Here's how the part is built. I have some questions about the finished solid (model axes, mm). A direction names the side the tool comes from. Give positions to 0.01 mm unless a question says otherwise; leave off trailing zeros. Loops run counter-clockwise (first coordinate to the right, second up) from the corner with the lowest first, then second, coordinate; pieces in that order, holes last. Notation, with made-up numbers: (55, 64.25) - (65, 64.25) arc R24 cw to (65, 95.25) - close; hole circle Ø11 at (73, -7). An arc over 180 degrees is marked (long way). Use a Markdown table: item, result.
Autodesk Inventor part; units mm, degrees
ref_plane "YZ Plane" through (0, 0, 0) normal (1, 0, 0) x (0, 1, 0)
ref_plane "XZ Plane" through (0, 0, 0) normal (0, 1, 0) x (-1, 0, 0)
ref_plane "XY Plane" through (0, 0, 0) normal (0, 0, 1) x (1, 0, 0)
sketch "Sketch1" plane through (0, 0, 0) normal (0, 0, 1) x (1, 0, 0)
  circle A0 centre (0, 0) radius 50
  circle A1 centre (0, 0) radius 35
  line L0 (-20, 45) -> (20, 45)
  line L1 (20, 45) -> (20, -75)
  line L2 (20, -75) -> (-20, -75)
  line L3 (-20, -75) -> (-20, 45)
  line L4 (-32.4459, -13.125) -> (-32.4459, -38.0429)
  line L5 (32.4459, -13.125) -> (32.4459, -38.0429)
  line L6 (-10, -67) -> (10, -67)
  line L7 (10, -67) -> (10, -64)
  line L8 (10, -64) -> (-10, -64)
  line L9 (-10, -64) -> (-10, -67)
  dimension "d0" = 100
  dimension "d1" = 70
  dimension "d4" = 40
  dimension "d5" = 120
  dimension "d9" = 20
  dimension "d10" = 3
extrude "Extrusion2" add sketch "Sketch1" along normal blind 5.5 contours A0 L5 A1 L1 L0 L3 L4 | L3 A1 L1 A0 | A0 L1 L2 L3 | L3 A1 L1 | L3 L0 L1 A1 | L9 L8 L7 L6
fillet "Fillet1" radius 8 2 edges at (20, -75, 2.75) (-20, -75, 2.75)
sketch "Sketch2" plane through (0, 0, 5.5) normal (0, 0, 1) x (1, 0, 0)
  line L0 (-10, -67) -> (10, -67)
  line L1 (10, -67) -> (10, -64)
  line L2 (10, -64) -> (-10, -64)
  line L3 (-10, -64) -> (-10, -67)
  point P0 (0, 0)
  dimension "d11" = 20
  dimension "d12" = 3
extrude "Extrusion3" cut sketch "Sketch2" against normal blind 5.5
sketch "Sketch4" plane through (0, 0, 5.5) normal (0, 0, 1) x (1, 0, 0)
  line L0 (39.75, 2.75) -> (45.25, 2.75)
  line L1 (45.25, 2.75) -> (45.25, -2.75)
  line L2 (45.25, -2.75) -> (39.75, -2.75)
  line L3 (39.75, -2.75) -> (39.75, 2.75)
  line L4 (-39.75, -2.75) -> (-45.25, -2.75)
  line L5 (-45.25, -2.75) -> (-45.25, 2.75)
  line L6 (-45.25, 2.75) -> (-39.75, 2.75)
  line L7 (-39.75, 2.75) -> (-39.75, -2.75)
  point P0 (0, 0)
  point P1 (0, 0)
  dimension "d24" = 5.5
  dimension "d25" = 5.5
  dimension "d26" = 360
extrude "Extrusion5" cut sketch "Sketch4" against normal blind 10
properties part number "central"
(1) We'd pull the mould along X, two halves only. Please class faces 4 (the face through (-17.719, -72.594, 2.788)), 5 (the face through (33.452, 10.293, 2.712)), 6 (the face through (-1.7, 49.97, 2.71)), 7 (the face through (32.446, -25, 3)): pulls with the +X half, pulls with the -X half, needs draft (parallel to the pull), parting line crosses it, or undercut.
A:
| item | result |
|---|---|
| face 4 | pulls with the -X half |
| face 5 | undercut |
| face 6 | parting line crosses it |
| face 7 | undercut |
(2) Suppose I cut it at B-B on x = 0. Write out the boundary of the cut face in (y, z), plus the area to 3 significant figures.
A:
| item | result |
|---|---|
| outline | (-75, 0) - (-67, 0) - (-67, 5.5) - (-75, 5.5) - close; (-64, 0) - (50, 0) - (50, 5.5) - (-64, 5.5) - close |
| area | 671 mm2 |
(3) On a 3-axis mill with a long thin cutter (end or side, diameter ignored), from which of +Z, -Z, +X, -X, +Y, -Y can I reach the whole of each face in a straight line? I mean faces 1 (the face through (0, -67, 3)), 2 (the face through (-20, -20, 3)), 3 (the face through (17.594, -72.719, 2.788)). Say none if no direction works.
A:
| item | result |
|---|---|
| face 1 | +Z, -Z |
| face 2 | +Z, -Z, -Y |
| face 3 | +Z, -Z, +X, -Y |
(4) Suppose I cut it at D-D on z = 4.6. Write out the boundary of the cut face in (x, y) (3 decimals).
A:
| item | result |
|---|---|
| outline | (-32.446, -38.043) - (-32.446, -13.125) arc R35 cw to (-20, 28.723) - (-20, -67) arc R8 ccw to (-12, -75) - (12, -75) arc R8 ccw to (20, -67) - (20, 28.723) arc R35 cw to (32.446, -13.125) - (32.446, -38.043) arc R50 ccw (long way) to start; hole (-45.25, -2.75) - (-39.75, -2.75) - (-39.75, 2.75) - (-45.25, 2.75) - close; hole (-10, -67) - (10, -67) - (10, -64) - (-10, -64) - close; hole (39.75, -2.75) - (45.25, -2.75) - (45.25, 2.75) - (39.75, 2.75) - close |
(5) Will these pins go through, and if not, where does the flat tip stop? pin 1 (12 mm diameter, centred on x = 2, y = -53.5, fed in from -Z); pin 2 (3 mm diameter, centred on x = 43, z = 2.5, fed in from -Y); pin 3 (3 mm diameter, centred on y = 32, z = 4.5, fed in from -X); pin 4 (2 mm diameter, centred on y = -18, z = 1.5, fed in from +X).
A:
| item | result |
|---|---|
| pin 1 | z = 0 |
| pin 2 | y = -27.89 |
| pin 3 | x = -39.62 |
| pin 4 | x = 47.02 |
(6) If I drill on line 1 (X direction, y = 18.5, z = 2.95); line 2 (X direction, y = -1, z = 5.25); line 3 (X direction, y = 28.5, z = 2.4), over which ranges is the centre line in solid material (lowest first)?
A:
| item | result |
|---|---|
| line 1 | -46.45 to -29.71, -20 to 20, 29.71 to 46.45 |
| line 2 | -49.99 to -45.25, -39.75 to -34.99, -20 to 20, 34.99 to 39.75, 45.25 to 49.99 |
| line 3 | -41.08 to -20.32, -20 to 20, 20.32 to 41.08 |
(7) Suppose I cut it at A-A on y = 0. Write out the boundary of the cut face in (x, z).
A:
| item | result |
|---|---|
| outline | (-50, 0) - (-45.25, 0) - (-45.25, 5.5) - (-50, 5.5) - close; (-39.75, 0) - (-35, 0) - (-35, 5.5) - (-39.75, 5.5) - close; (-20, 0) - (20, 0) - (20, 5.5) - (-20, 5.5) - close; (35, 0) - (39.75, 0) - (39.75, 5.5) - (35, 5.5) - close; (45.25, 0) - (50, 0) - (50, 5.5) - (45.25, 5.5) - close |
(8) Suppose I cut it at C-C on y = 27. Write out the boundary of the cut face in (x, z).
A:
| item | result |
|---|---|
| outline | (-42.08, 0) - (-22.27, 0) - (-22.27, 5.5) - (-42.08, 5.5) - close; (-20, 0) - (20, 0) - (20, 5.5) - (-20, 5.5) - close; (22.27, 0) - (42.08, 0) - (42.08, 5.5) - (22.27, 5.5) - close |
